Build history of the part. All positions in model axes, mm. Face numbers are marked on the shaded views. A direction names the side the tool comes from. Give positions to 0.01 mm unless a question says otherwise; leave off trailing zeros. Loops run counter-clockwise (first coordinate to the right, second up) from the corner with the lowest first, then second, coordinate; pieces in that order, holes last. Notation, with made-up numbers: M 37.5,10.5 L 95.5,10.5 A20 cw 95.5,43.5 Z; hole C 44.25,19.25 d3. An arc over 180 degrees is marked long. Put each result on its own line as item: value.
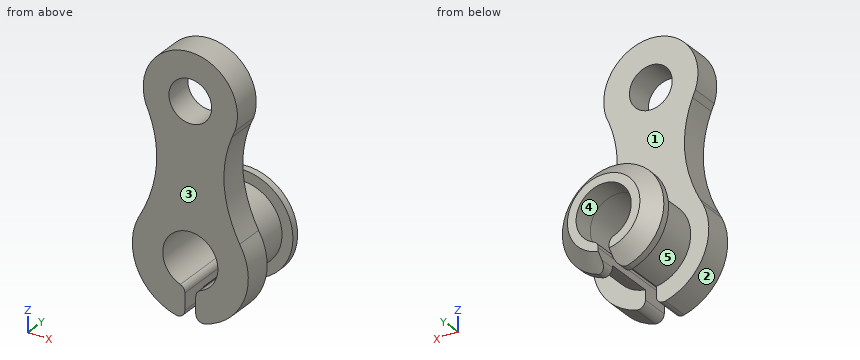
Autodesk Inventor part; units mm, degrees
ref_plane "YZ Plane" through (0, 0, 0) normal (1, 0, 0) x (0, 1, 0)
ref_plane "XZ Plane" through (0, 0, 0) normal (0, 1, 0) x (-1, 0, 0)
ref_plane "XY Plane" through (0, 0, 0) normal (0, 0, 1) x (1, 0, 0)
sketch "Sketch1" plane through (0, 0, 0) normal (0, 1, 0) x (-1, 0, 0)
  circle A0 centre (0, 0) radius 2.95
  circle A1 centre (0, 0) radius 6.5
  circle A2 centre (0, -21) radius 8
  spline S0 degree 2 poles (6.1434, -2.1233) (2.6668, -9.5534) (7.2026, -17.5183) knots 0 0 0 1 1 1
  line L0 (0, 0) -> (0, -21) construction
  spline S1 degree 2 poles (-6.1434, -2.1233) (-2.6668, -9.5534) (-7.2026, -17.5183) knots 0 0 0 1 1 1
  point P0 (4.6554, -9.4486)
  point P1 (-4.6554, -9.4486)
  point P2 (-6.1434, -2.1233)
  point P3 (-6.812, -16.8052)
  dimension "d1" = 13
  dimension "d2" = 16
  dimension "d0" = 5.9
  dimension "d3" = 21
extrude "Extrusion1" add sketch "Sketch1" along normal blind 4 contours A1 S0 S1 | A1 S0 A2 S1 | S1 A2 | A2 S0 S1
sketch "Sketch2" plane through (0, 4, 0) normal (0, 1, 0) x (1, 0, 0)
  arc A0 (6.812, 16.8052) -> (-7.2026, 17.5183) centre (0, 21) ccw
  arc A1 (-6.1434, 2.1233) -> (6.1434, 2.1233) centre (0, 0) ccw
  circle A2 centre (0, 0) radius 2.95
  circle A3 centre (0, 21) radius 5.5
  line L0 (0.75, 12.2819) -> (-0.75, 12.2819)
  line L1 (-0.75, 12.2819) -> (-0.75, 29.7181)
  line L2 (-0.75, 29.7181) -> (0.75, 29.7181)
  line L3 (0.75, 29.7181) -> (0.75, 12.2819)
  line L4 (0.75, 12.2819) -> (-0.75, 29.7181) construction
  line L5 (-0.75, 12.2819) -> (0.75, 29.7181) construction
  circle A4 centre (0, 21) radius 3.8038
  point P0 (0.75, 26.4486)
  point P1 (0.75, 15.5514)
  point P2 (-0.75, 15.5514)
  point P3 (-0.75, 26.4486)
  point P4 (-0.75, 24.7291)
  point P5 (0.75, 24.7291)
  dimension "d6" = 11
  dimension "d7" = 1.5
extrude "Extrusion2" cut sketch "Sketch2" against normal blind 5 contours L3 A3 L1 A0 | A0 L1 L2 L3 | L3 A4 L1 A3 | A4 L3 | L3 A4 L1 | L1 A4 picked at (-0.5838, 25.3244)
extrude "Extrusion3" add sketch "Sketch2" along normal blind 7 contours A3 L3 A4 | L1 A4 A3 | L1 A4 L3 A3 picked at (-0.5838, 16.6756)
sketch "Sketch4" plane through (0, 11, 0) normal (0, 1, 0) x (1, 0, 0)
  line L0 (-0.75, 24.7291) -> (-0.75, 26.4486)
  arc A0 (-0.75, 26.4486) -> (0.75, 26.4486) centre (0, 21) ccw
  line L1 (0.75, 26.4486) -> (0.75, 24.7291)
  arc A1 (-0.75, 24.7291) -> (0.75, 24.7291) centre (0, 21) ccw
  circle A2 centre (0, 21) radius 5.5
  circle A3 centre (0, 21) radius 3.8038
  circle A4 centre (0, 21) radius 7
  line L2 (-0.75, 12.2819) -> (-0.75, 29.7181)
  line L3 (0.75, 29.7181) -> (0.75, 12.2819)
  point P0 (0, 0)
  point P1 (0.75, 27.9597)
  point P2 (-0.75, 27.9597)
  dimension "d12" = 1.5
extrude "Extrusion4" add sketch "Sketch4" along normal blind 3 contours A1 L2 A0 L0 | A0 L2 A4 | A1 L3 A0 L2 | L1 A0 L3 A1 | A0 L3 A4 L2 | L3 A4 A0
chamfer "Chamfer1" distance 2 angle 45 1 edges at (0, 14, -14)
fillet "Fillet1" radius 1 8 edges at (0.75, 2, -28.9648) (-0.75, 2, -28.9648) (0.75, 12.5, -24.7291) (0.75, 2, -24.7291) (-0.75, 12.5, -24.7291) (-0.75, 2, -24.7291) (0.75, 11.5, -27.9597) (-0.75, 11.5, -27.9597)
properties part number "Servo_Pulley"
Q1. Slice it at B-B (x = 0). List the corners of the cut face in (y, z).
Here are the results:
outline: M 0,-17.2 L 14,-17.2 L 14,-16 L 12,-14 L 11,-14 L 11,-15.5 L 4,-15.5 L 4,-2.95 L 0,-2.95 Z; M 0,2.95 L 4,2.95 L 4,6.5 L 0,6.5 Z
Q2. Slice it at D-D (z = -21). List the corners of the cut face in (x, y), and give its area (3 significant figures).
Here are the results:
outline: M -8,0 L -3.8,0 L -3.8,14 L -5,14 L -7,12 L -7,11 L -5.5,11 L -5.5,4 L -8,4 Z; M 3.8,0 L 8,0 L 8,4 L 5.5,4 L 5.5,11 L 7,11 L 7,12 L 5,14 L 3.8,14 Z
area: 72.5 mm²
Q3. Probe line 1 (Z direction, x = 0, y = 2.25); line 2 (Y direction, x = -1, z = -9); line 3 (Z direction, x = -3, y = 11.5). List the from-to ranges inside material, lowest first. Write a range as from..to.
Here are the results:
line 1: -17.2..-2.95, 2.95..6.5
line 2: 0..4
line 3: -27.32..-23.34, -18.66..-14.68
Q4. Mould opens along Y. For the marked faces 1, 2 and 3 say: pulls with the +Y half, pulls with the -Y half, needs draft (parallel to the pull), parting line crosses it, or undercut.
Here are the results:
face 1: undercut
face 2: needs draft
face 3: pulls with the -Y half
Q5. Slice it at C-C (y = 9.5). List the corners of the cut face in (x, z).
Here are the results:
outline: M -1.39,-24.54 A3.8 cw long 1.39,-24.54 A1 ccw 0.75,-25.47 L 0.75,-26.45 A5.5 ccw long -0.75,-26.45 L -0.75,-25.47 A1 ccw Z
Q6. Tool access for the marked faces 4 and 5: list every direction of +Z, -Z, +X, -X, +Y, -Y with a clear straight run to the whole face (end or side of a thin tool).
Here are the results:
face 4: +Y, -Y
face 5: none
Q7. Drop flat-ended pins along their axis: pin 1 Ø1.5 at (y, z) = (6.5, -24.5) entering from -X; pin 2 Ø8 at (x, z) = (-3, 2) entering from +Y; pin 3 Ø2.5 at (y, z) = (8.5, -26.5) entering from +X; pin 4 Ø7 at (x, z) = (0, -21) entering from -Y. Give the stop position or say it passes through.
Here are the results:
pin 1: x = -4.76
pin 2: y = 4
pin 3: x = 3.49
pin 4: through
Q8. Slice it at A-A (z = 0). List the corners of the cut face in (x, y), and give its area (3 significant figures).
Here are the results:
outline: M -6.5,0 L -2.95,0 L -2.95,4 L -6.5,4 Z; M 2.95,0 L 6.5,0 L 6.5,4 L 2.95,4 Z
area: 28.4 mm²
